Can you work these out from the model? Positions are in its coordinate system, mm. Face numbers are marked on the shaded views. A direction names the side the tool comes from. Round coordinates to 2 decimals unless told otherwise and drop trailing zeros. Loops run counter-clockwise (first coordinate to the right, second up) from the corner with the lowest first, then second, coordinate; pieces in that order, holes last. Notation, with made-up numbers: (14, 68.5) - (34, 68.5) arc R16 cw to (34, 75.5) - close; hole circle Ø6 at (-4.75, 49.5). An arc over 180 degrees is marked (long way). Answer as CSV lines item,"result".
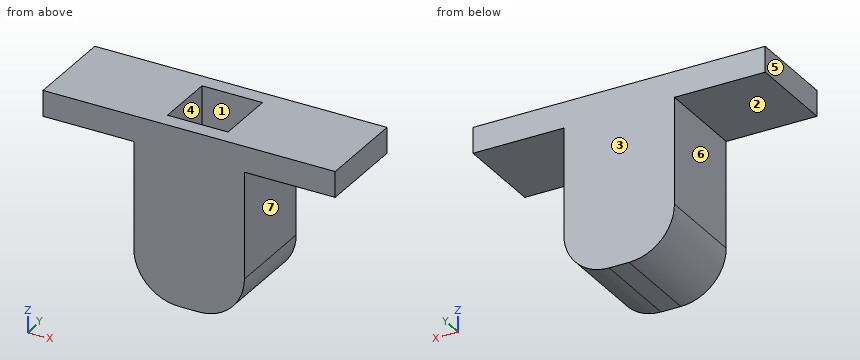
```python
from build123d import *

# Parameters (mm, degrees)
BOSS_EXTRUDE1_DEPTH = 3
SKETCH3_W           = 2
SKETCH3_H           = 2
CUT_EXTRUDE1_DEPTH  = 5


with BuildPart() as part:
    # Sketch1 → Boss-Extrude1 (new body)
    with BuildSketch(Plane(origin=(0, 0, 0), x_dir=(1, 0, 0), z_dir=(0, 1, 0))):
        with BuildLine():
            Line((4.222106341, 0), (4.222106341, 0.85))
            Line((4.222106341, 0.85), (7.222106341, 0.85))
            Line((7.222106341, 0.85), (7.222106341, 4.357735156))
            ThreePointArc((7.222106341, 4.357735156), (7.661446169, 5.418395328), (8.722106341, 5.857735156))
            Line((8.722106341, 5.857735156), (9.380074809, 5.857735156))
            ThreePointArc((9.380074809, 5.857735156), (10.44073498, 5.418395328), (10.880074809, 4.357735156))
            Line((10.880074809, 4.357735156), (10.880074809, 0.85))
            Line((10.880074809, 0.85), (13.880074809, 0.85))
            Line((13.880074809, 0.85), (13.880074809, 0))
            Line((13.880074809, 0), (4.222106341, 0))
        make_face()
    extrude(amount=BOSS_EXTRUDE1_DEPTH)

    # Sketch3 → Cut-Extrude1 (cut)
    with BuildSketch(Plane.XY):
        with Locations((9.051090575, 1.5)):
            Rectangle(SKETCH3_W, SKETCH3_H)
    extrude(amount=-CUT_EXTRUDE1_DEPTH, mode=Mode.SUBTRACT)


solid = part.part
```
Q1. Imagine slicing it at A-A (z = -1.3). Write out the boundary of the cut face in (x, y), then the cut area to 3 significant figures.
Checks:
outline,"(7.22, 0) - (10.88, 0) - (10.88, 3) - (7.22, 3) - close; hole (8.05, 0.5) - (10.05, 0.5) - (10.05, 2.5) - (8.05, 2.5) - close"
area,"6.97 mm²"
Q2. On a 3-axis mill with a long thin cutter (end or side, diameter ignored), from which of +Z, -Z, +X, -X, +Y, -Y can I reach the whole of each face in a straight line? I mean the marked faces 5, 6 and 7. Say none if no direction works.
Checks:
face 5,"+Z, -Z, -X, +Y, -Y"
face 6,"-Z, -X, +Y, -Y"
face 7,"-Z, +X, +Y, -Y"
Q3. We'd pull the mould along Y, two halves only. Please class the marked faces 1, 2, 3 and 4: pulls with the +Y half, pulls with the -Y half, needs draft (parallel to the pull), parting line crosses it, or undercut.
Checks:
face 1,"undercut"
face 2,"needs draft"
face 3,"pulls with the +Y half"
face 4,"undercut"
Q4. I'm going to push flat-ended pins straight in: pin 1 Ø1.5 at (y, z) = (1.5, -3) entering from +X; pin 2 Ø2 at (x, z) = (12.5, -3.5) entering from +Y (1 decimal); pin 3 Ø0.6 at (x, y) = (9, 1.5) entering from +Z; pin 4 Ø1.5 at (x, y) = (5.5, 1) entering from -Z. Where does each tip first touch, or does it pass through?
Checks:
pin 1,"x = 10.88"
pin 2,"through"
pin 3,"z = -5"
pin 4,"z = -0.85"
Q5. Imagine slicing it at D-D (y = 2.8). Write out the boundary of the cut face in (x, z), then the cut area to 3 significant figures.
Checks:
outline,"(4.22, -0.85) - (7.22, -0.85) - (7.22, -4.36) arc R1.5 ccw to (8.72, -5.86) - (9.38, -5.86) arc R1.5 ccw to (10.88, -4.36) - (10.88, -0.85) - (13.88, -0.85) - (13.88, 0) - (4.22, 0) - close"
area,"25.6 mm²"
Q6. If I drill on line 1 along Y through (x, z) = (10, -2.6); line 2 along X through (y, z) = (0.9, -1.6); line 3 along Z through (x, y) = (8.75, 0.95), over which ranges is the centre line in solid material (lowest first)? Write a range as [from, to].
Checks:
line 1,"[0, 0.5], [2.5, 3]"
line 2,"[7.22, 8.05], [10.05, 10.88]"
line 3,"[-5.86, -5]"
Q7. Imagine slicing it at C-C (x = 9). Write out the boundary of the cut face in (y, z), then the cut area to 3 significant figures.
Checks:
outline,"(0, -5.86) - (3, -5.86) - (3, 0) - (2.5, 0) - (2.5, -5) - (0.5, -5) - (0.5, 0) - (0, 0) - close"
area,"7.57 mm²"
Q8. Imagine slicing it at B-B (y = 0.75). Write out the boundary of the cut face in (x, z).
Checks:
outline,"(4.22, -0.85) - (7.22, -0.85) - (7.22, -4.36) arc R1.5 ccw to (8.72, -5.86) - (9.38, -5.86) arc R1.5 ccw to (10.88, -4.36) - (10.88, -0.85) - (13.88, -0.85) - (13.88, 0) - (10.05, 0) - (10.05, -5) - (8.05, -5) - (8.05, 0) - (4.22, 0) - close"
